```python
from build123d import *

# Parameters (mm, degrees)
BOSS_EXTRUDE1_DEPTH = 50
FILLET1_R           = 22


with BuildPart() as part:
    # Sketch1 → Boss-Extrude1 (new body)
    with BuildSketch(Plane(origin=(0, 0, 0), x_dir=(1, 0, 0), z_dir=(0, 1, 0))):
        with BuildLine():
            ThreePointArc((-56.848272026, 73.599801144), (-28.960885768, 65.300905733), (0, 62.5))
            ThreePointArc((0, 62.5), (28.960885768, 65.300905733), (56.848272026, 73.599801144))
            ThreePointArc((56.848272026, 73.599801144), (100, 65), (109.144044644, 21.960313031))
            ThreePointArc((109.144044644, 21.960313031), (106.045073596, 11.173947987), (105, 0))
            ThreePointArc((105, 0), (106.045073596, -11.173947987), (109.144044644, -21.960313031))
            ThreePointArc((109.144044644, -21.960313031), (100, -65), (56.848272026, -73.599801144))
            ThreePointArc((56.848272026, -73.599801144), (28.960885768, -65.300905733), (0, -62.5))
            ThreePointArc((0, -62.5), (-28.960885768, -65.300905733), (-56.848272026, -73.599801144))
            ThreePointArc((-56.848272026, -73.599801144), (-100, -65), (-109.144044644, -21.960313031))
            ThreePointArc((-109.144044644, -21.960313031), (-106.045073596, -11.173947987), (-105, 0))
            ThreePointArc((-105, 0), (-106.045073596, 11.173947987), (-109.144044644, 21.960313031))
            ThreePointArc((-109.144044644, 21.960313031), (-100, 65), (-56.848272026, 73.599801144))
        make_face()
    extrude(amount=BOSS_EXTRUDE1_DEPTH)

    # Fillet1
    fillet1_edges = [part.edges().sort_by_distance(p)[0] for p in [
        (0, 0, 62.5),
        (-100, 0, 65),
        (105, 50, 0),
        (-105, 0, 0),
        (-100, 0, -65),
        (0, 0, -62.5),
        (100, 0, -65),
        (105, 0, 0),
        (100, 0, 65),
        (100, 50, -65),
        (0, 50, -62.5),
        (-100, 50, -65),
        (-105, 50, 0),
        (-100, 50, 65),
        (0, 50, 62.5),
        (100, 50, 65),
    ]]
    fillet(fillet1_edges, radius=FILLET1_R)


solid = part.part
```
CAD build for the part. Positions are in the model's coordinates, mm. Coordinates: 2 decimals unless noted, no trailing zeros. Loops run counter-clockwise (first coordinate to the right, second up) from the corner with the lowest first, then second, coordinate; pieces in that order, holes last. Notation, with made-up numbers: (14, 86.25) - (18, 86.25) arc R9 cw to (18, 102.25) - close; hole circle Ø11 at (66.25, -25). An arc over 180 degrees is marked (long way). Return JSON: item names as keys, results as strings.
1. Drop flat-ended pins along their axis: pin 1 (10 mm diameter, centred on x = -42, y = 39.5, fed in from +Z); pin 2 (2 mm diameter, centred on y = 40, z = -51.5, fed in from -X); pin 3 (1 mm diameter, centred on y = 42, z = -19.5, fed in from +X). Give the stop position or say it passes through.
Result:
{"pin 1": "stops at z = 67.98", "pin 2": "stops at x = -105.93", "pin 3": "stops at x = 103.4"}
2. Probe L1, parallel to X at y = 4.5, z = 18; L2, parallel to Z at x = -40, y = 8.5; L3, parallel to Y at x = -102.5, z = 17. List the from-to ranges inside material, lowest first. Write a range as from..to.
Result:
{"L1": "x = -98.72..98.72", "L2": "z = -63.09..63.09", "L3": "y = 8.33..41.67"}
3. Band-saw the part on A-A (y = 25.5). Give the cut face in (x, z), and give its area (3 significant figures).
Result:
{"outline": "(-109.14, -21.96) arc R40 ccw to (-56.85, -73.6) arc R151.13 cw to (56.85, -73.6) arc R40 ccw to (109.14, -21.96) arc R60.26 cw to (109.14, 21.96) arc R40 ccw to (56.85, 73.6) arc R151.13 cw to (-56.85, 73.6) arc R40 ccw to (-109.14, 21.96) arc R60.26 cw to start", "area": "29,900 mm2"}
